Part model, mm, in its own coordinate system. A direction names the side the tool comes from. Coordinates: 2 decimals unless noted, no trailing zeros. Write each loop counter-clockwise with the first axis right and the second up, starting at its lowest first coordinate (ties: lowest second). Pieces come first, ordered by that corner, then holes. Notation, with made-up numbers: M -11.75,37.25 L 39.25,37.25 A14 ccw 39.25,61.25 Z; hole C -7.75,87 d3. An arc over 180 degrees is marked long. Use a Markdown table: item, result. Add a question column.
Q1. Slice it at A-A on z = 55. Write the cut outline in (x, y).
Q2. Slice it at C-C on x = -26.5. Write the cut outline in (y, z).
Q3. Tool access for faces 1 (the flat face through (-2, 1, 64)), 2 (the flat face through (-5, 29, 17)), 3 (the cylindrical face through (-4.014, 54.635, 16.69)): list every direction of +Z, -Z, +X, -X, +Y, -Y with a clear straight run to the whole face (end or side of a thin tool).
Q4. Slice it at B-B on z = 6. Write the cut outline in (x, y), then the cut area to 4 significant figures.
Q5. Mould opens along X. For faces 4 (the flat face through (-2, 68, 27)), 5 (the cylindrical face through (-12.5, 1.23, 6.07)), 6 (the flat face through (-3, 15, 71)) say: released by +X, released by -X, zero draft, split by the parting line, or undercut.
Q6. Wall check: L1, parallel to Z at x = -42, y = 1; L2, parallel to Z at x = -26.5, y = 1; L3, parallel to Z at x = -2.3, y = 60. Give the ranges that are in metal, low to high. Write a range as from..to.
Q7. Slice it at D-D on y = 14.5. Write the cut outline in (x, z), then the cut area to 3 significant figures.
Q8. Pin check, flat tips, straight feed: pin 1 Ø4 at (x, z) = (-11, 6) entering from -Y; pin 2 Ø5.5 at (y, z) = (12, 72.5) entering from -X; pin 3 Ø5 at (x, y) = (-17.5, 9) entering from +Z; pin 4 Ø4 at (y, z) = (60, 15) entering from +X. Stop position of each tip, or through.
from build123d import *

# Parameters (mm, degrees)
F0_W           = 48
F0_H           = 43
F0_R           = 1.5
F0_R_2         = 12.5
F1_DEPTH       = 2.5
F3_DEPTH       = 5
F5_D           = 6.6
F5_DEPTH       = 20
F5_CBORE_D     = 11.25
F5_CBORE_DEPTH = 2
F7_DEPTH       = 4
F8_DEPTH       = 1


with BuildPart() as f1:
    # F0 (on Front) → F1 (new body)
    with BuildSketch(Plane.XZ):
        with Locations((-24, 21.5)):
            Rectangle(F0_W, F0_H)
        with Locations((-42, 6)):
            Circle(F0_R, mode=Mode.SUBTRACT)
        with Locations((-11, 6)):
            Circle(F0_R, mode=Mode.SUBTRACT)
        with Locations((-26.5, 21.5)):
            Circle(F0_R_2, mode=Mode.SUBTRACT)
        with Locations((-42, 37)):
            Circle(F0_R, mode=Mode.SUBTRACT)
    extrude(amount=-F1_DEPTH)

    # F2 (on Right) → F3 (join)
    with BuildSketch(Plane.YZ):
        Polygon((1, 43), (0, 43), (0, 0), (65, 0), (70, 5), (70, 25), (65, 30), (40, 30), (30, 40), (30, 80.5), (25.5, 85), (5.5, 85), (1, 80.5), align=None)
    extrude(amount=-F3_DEPTH)

    # F5
    with Locations(Plane(origin=(-5, 0, 0), x_dir=(0, -1, 0), z_dir=(-1, 0, 0))):
        with Locations((-14.795874, 75), (-14.795874, 55), (-60, 15)):
            CounterBoreHole(F5_D / 2, F5_CBORE_D / 2, F5_CBORE_DEPTH, depth=F5_DEPTH)

    # F6 (on face) → F7 (join)
    with BuildSketch(Plane.XY.offset(43)):
        Polygon((-5, 30), (-48, 2.5), (-5, 2.5), (-5, 1), (0, 1), (0, 30), align=None)
        Polygon((-48, 2.5), (-48, 0), (0, 0), (0, 1), (-5, 1), (-5, 2.5), align=None)
    extrude(amount=F7_DEPTH)

    # F7_face (on face) → F8 (cut)
    with BuildSketch(Plane(origin=(-19.333333, 11.666667, 43), x_dir=(1, 0, 0), z_dir=(0, 0, -1))):
        Polygon((14.333333, -18.333333), (14.333333, 9.166667), (-28.666667, 9.166667), align=None)
    extrude(amount=-F8_DEPTH, mode=Mode.SUBTRACT)


solid = f1.part
Recorded:
| question | item | result |
|---|---|---|
| 1 | outline | M -5,1 L 0,1 L 0,11.5 L -3,11.5 L -3,9.17 L -5,9.17 Z; M -5,20.42 L -3,20.42 L -3,18.1 L 0,18.1 L 0,30 L -5,30 Z |
| 2 | outline | M 0,0 L 2.5,0 L 2.5,9 L 0,9 Z; M 0,34 L 2.5,34 L 2.5,44 L 16.25,44 L 16.25,47 L 0,47 Z |
| 3 | face 1 | +Z, +X, -X, -Y |
| 3 | face 2 | -Z, -X, +Y |
| 3 | face 3 | -X |
| 4 | outline | M -48,0 L -43.5,0 L -43.5,2.5 L -48,2.5 Z; M -40.5,0 L -12.5,0 L -12.5,2.5 L -40.5,2.5 Z; M -9.5,0 L 0,0 L 0,70 L -5,70 L -5,2.5 L -9.5,2.5 Z |
| 4 | area | 442.5 mm² |
| 5 | face 4 | zero draft |
| 5 | face 5 | undercut |
| 5 | face 6 | released by -X |
| 6 | L1 | 0..4.5, 7.5..35.5, 38.5..47 |
| 6 | L2 | 0..9, 34..47 |
| 6 | L3 | 0..11.7, 18.3..30 |
| 7 | outline | M -29.24,44 L -5,44 L -5,0 L 0,0 L 0,51.71 L -3,51.71 L -3,49.38 L -5,49.38 L -5,47 L -29.24,47 Z; M -5,60.62 L -3,60.62 L -3,58.29 L 0,58.29 L 0,71.71 L -3,71.71 L -3,69.38 L -5,69.38 Z; M -5,80.62 L -3,80.62 L -3,78.29 L 0,78.29 L 0,85 L -5,85 Z |
| 7 | area | 413 mm² |
| 8 | pin 1 | y = 0 |
| 8 | pin 2 | x = -5 |
| 8 | pin 3 | z = 47 |
| 8 | pin 4 | through |
